```python
from build123d import *

# Parameters (mm, degrees)
SKETCH1_W                    = 45
SKETCH1_H                    = 26
BOSS_EXTRUDE5_DEPTH          = 3
BOSS_EXTRUDE6_DEPTH          = 14
CUT_EXTRUDE1_DEPTH           = 30.516944286
CUT_EXTRUDE1_DEPTH_BACK      = 30.516944286
SKETCH9_W                    = 15
SKETCH9_H                    = 20
M2_CLEARANCE_HOLE2_OUTLINE_R = 1.1
M2_CLEARANCE_HOLE2_DEPTH     = 3
M2_CLEARANCE_HOLE3_D         = 2.2
FILLET1_R                    = 1.5
FILLET2_R                    = 1.5


# Read off the part's stored shape, not the designer's step: M2 Clearance Hole2
with BuildPart() as part:
    # Sketch1 → Boss-Extrude5 (new body)
    with BuildSketch(Plane.XY):
        Rectangle(SKETCH1_W, SKETCH1_H)
    extrude(amount=BOSS_EXTRUDE5_DEPTH)

    # Sketch8 → Boss-Extrude6 (add)
    with BuildSketch(Plane.XY.offset(3)):
        Polygon((-9.931802589, -10), (-9.931802589, 13), (-12.931802589, 13), (-12.931802589, -13), (13.068197411, -13), (13.068197411, 13), (10.068197411, 13), (10.068197411, -10), align=None)
    extrude(amount=BOSS_EXTRUDE6_DEPTH)

    # Sketch9 → Cut-Extrude1 (cut, two sides: drawn at the far end of the back side and taken through both)
    with BuildSketch(Plane.XY.offset(3).offset(-CUT_EXTRUDE1_DEPTH_BACK)):
        with Locations((0.068197411, 3)):
            Rectangle(SKETCH9_W, SKETCH9_H)
    extrude(amount=CUT_EXTRUDE1_DEPTH + CUT_EXTRUDE1_DEPTH_BACK, mode=Mode.SUBTRACT)

    # M2 Clearance Hole2 outline → M2 Clearance Hole2 (cut)
    with BuildSketch(Plane.XY):
        with Locations((17.5, 8)):
            Circle(M2_CLEARANCE_HOLE2_OUTLINE_R)
        with Locations((-17.5, -8)):
            Circle(M2_CLEARANCE_HOLE2_OUTLINE_R)
        with Locations((-17.5, 8)):
            Circle(M2_CLEARANCE_HOLE2_OUTLINE_R)
        with Locations((17.5, -8)):
            Circle(M2_CLEARANCE_HOLE2_OUTLINE_R)
    extrude(amount=M2_CLEARANCE_HOLE2_DEPTH, mode=Mode.SUBTRACT)

    # M2 Clearance Hole3 (through all)
    with Locations(Plane.ZY.offset(12.931802589)):
        with Locations((13, 2.5)):
            Hole(M2_CLEARANCE_HOLE3_D / 2)

    # Fillet1
    fillet1_edges = [part.edges().sort_by_distance(p)[0] for p in [
        (-22.5, 0, 3),
        (-17.715901295, 13, 3),
        (17.784098705, -13, 3),
        (-17.715901295, -13, 3),
        (-12.931802589, 0, 3),
        (-12.931802589, 13, 10),
        (-12.931802589, -13, 10),
        (13.068197411, 0, 3),
        (13.068197411, -13, 10),
        (13.068197411, 13, 10),
        (-12.931802589, 0, 17),
        (0.068197411, -13, 17),
        (13.068197411, 0, 17),
        (0.068197411, -10, 17),
        (22.5, 0, 3),
        (17.784098705, 13, 3),
    ]]
    fillet(fillet1_edges, radius=FILLET1_R - 0.0001)  # a hair under: the kernel refuses the full size

    # Fillet2
    fillet2_edges = [part.edges().sort_by_distance(p)[0] for p in [
        (8.818197411, 13, 3),
        (-8.681802589, 13, 3),
        (7.568197411, 3, 3),
        (0.068197411, -7, 3),
        (-7.431802589, 3, 3),
        (-7.431802589, 13, 1.5),
        (7.568197411, 13, 1.5),
    ]]
    fillet(fillet2_edges, radius=FILLET2_R)


solid = part.part
```
Input: part model. Units: mm. Frame: model coordinates. A direction names the side the tool comes from. Give positions to 0.01 mm unless a question says otherwise; leave off trailing zeros. Order: outer loops, then holes, each group sorted by start corner. A loop starts at its lowest first (then second) coordinate and runs counter-clockwise, first axis right, second up. Notation, with made-up numbers: M -36.75,86 L 21.25,86 A27 cw 21.25,102 Z; hole C -20,6 d3. An arc over 180 degrees is marked long. Return JSON: item names as keys, results as strings.
Item 1: Cut plane A-A (y = 2.5). State how many separate pieces and enclosed holes the cut face has, then the cut area to 3 significant figures.
Solutions:
{"separate pieces": "4", "enclosed holes": "0", "area": "159 mm^2"}
Item 2: Ray query, probe 1 along Y at (x, z) = (-17.5, 1.5); probe 2 along X at (y, z) = (9.25, 4.75); probe 3 along Y at (x, z) = (-17.5, 2). Return the intervals inside material, ascending.
Solutions:
{"probe 1": "-13 to -9.1, -6.9 to 6.9, 9.1 to 13", "probe 2": "-12.93 to -9.93, 10.07 to 13.07", "probe 3": "-12.91 to -9.1, -6.9 to 6.9, 9.1 to 12.91"}
Item 3: Cut plane C-C (z = 13). Return loops of the section in (x, y), then the cut area to 3 significant figures.
Solutions:
{"outline": "M -12.93,-11.5 A1.5 ccw -11.43,-13 L 11.57,-13 A1.5 ccw 13.07,-11.5 L 13.07,1.4 L 10.07,1.4 L 10.07,-10 L -9.93,-10 L -9.93,1.4 L -12.93,1.4 Z; M -12.93,3.6 L -9.93,3.6 L -9.93,13 L -11.43,13 A1.5 ccw -12.93,11.5 Z; M 10.07,3.6 L 13.07,3.6 L 13.07,11.5 A1.5 ccw 11.57,13 L 10.07,13 Z", "area": "201 mm^2"}
Item 4: Access query for faces 1 (the cylindrical face through (7.996, 12.549, 0.761)), 2 (the cylindrical face through (18.59, 12.55, 2.57)), 3 (the cylindrical face through (-9.42, 12.57, 2.55)), 4 (the cylindrical face through (18.59, -12.57, 2.55)), 5 (the cylindrical face through (-18.41, -12.57, 2.55)). Directions: +Z, -Z, +X, -X, +Y, -Y. A direction counts if a zero-diameter tool reaches every point of the face in a straight line with its end or side. Return the directions, or none.
Solutions:
{"face 1": "+Z, -Z, +Y", "face 2": "+Z, +X, +Y", "face 3": "+Z, +Y", "face 4": "+Z, +X, -Y", "face 5": "+Z, -X, -Y"}
Item 5: Pull-direction query (Z, two-part tool) for faces 6 (the cylindrical face through (-11.41, 1.83, 13.87)), 7 (the flat face through (13.068, 0, 10)), 8 (the flat face through (0, -8, 0)), 9 (the cylindrical face through (13.496, 0.161, 3.451)); classes: +Z half, -Z half, draft (parallel to the pull), parting line (faces both ways), or undercut.
Solutions:
{"face 6": "undercut", "face 7": "draft", "face 8": "-Z half", "face 9": "+Z half"}
Item 6: Cut plane D-D (z = 1). Return loops of the section in (x, y).
Solutions:
{"outline": "M -22.5,-13 L 22.5,-13 L 22.5,13 L 9.07,13 A1.5 ccw 7.57,11.5 L 7.57,-7 L -7.43,-7 L -7.43,11.5 A1.5 ccw -8.93,13 L -22.5,13 Z; hole C -17.5,-8 d2.2; hole C -17.5,8 d2.2; hole C 17.5,-8 d2.2; hole C 17.5,8 d2.2"}
Item 7: First-contact query: P1, Ø5.5, axis at x = -16.5, y = 5.5, coming from the +Z side; P2, Ø3.5, axis at y = -1.5, z = 8, coming from the +X side; P3, Ø8, axis at y = -3.5, z = 8.5, coming from the -X side; P4, Ø8, axis at x = 11, y = 10, coming from the -Z side. Flat tips, straight axial feed; report the tip coordinate or a pass-through.
Solutions:
{"P1": "z = 3.16", "P2": "x = 13.07", "P3": "x = -12.93", "P4": "z = 0"}
Item 8: Cut plane B-B (x = -17.5). Return loops of the section in (y, z), then the cut area to 3 significant figures.
Solutions:
{"outline": "M -13,0 L -9.1,0 L -9.1,3 L -11.5,3 A1.5 ccw -13,1.5 Z; M -6.9,0 L 6.9,0 L 6.9,3 L -6.9,3 Z; M 9.1,0 L 13,0 L 13,1.5 A1.5 ccw 11.5,3 L 9.1,3 Z", "area": "63.8 mm^2"}
